Can you work these out from the drawing? Everything is in mm from the part's minimum corner. A direction names the side the tool comes from. Coordinates: 2 decimals unless noted, no trailing zeros. Loops run counter-clockwise (first coordinate to the right, second up) from the corner with the lowest first, then second, coordinate; pieces in that order, holes last.
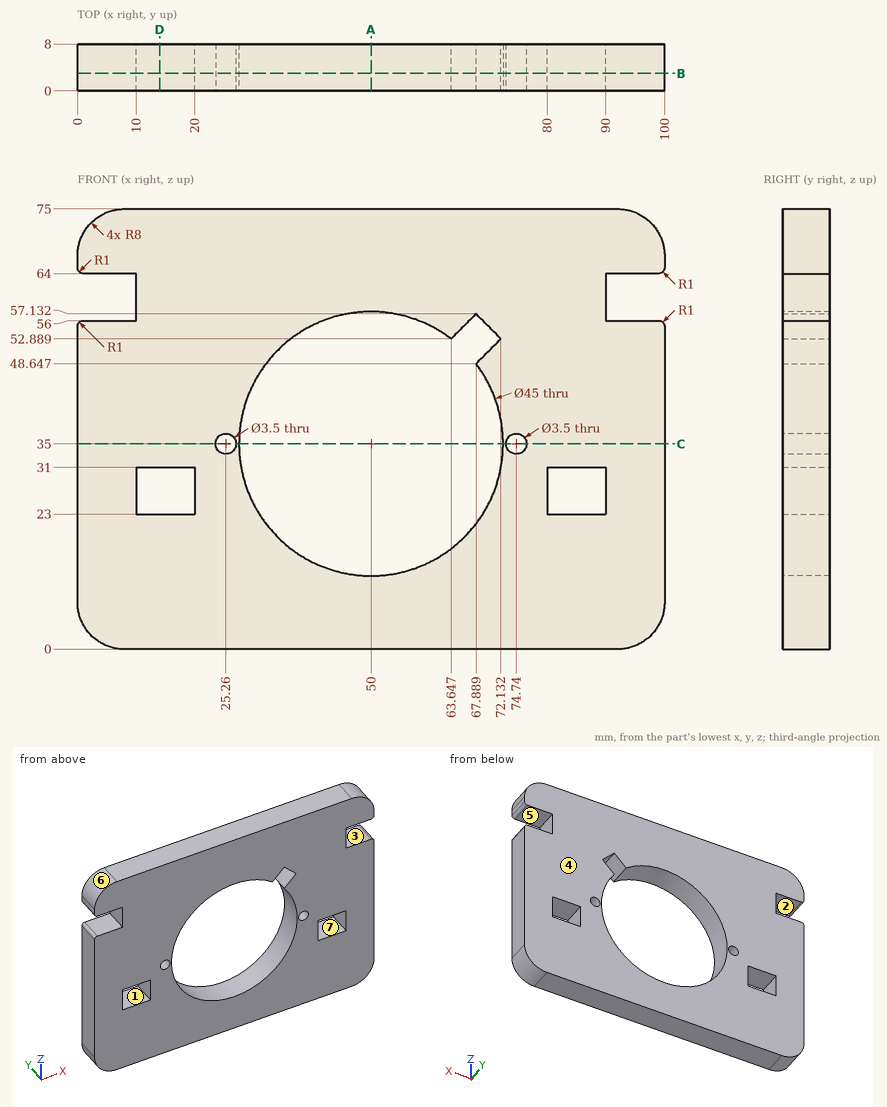
Item 1: On a 3-axis mill with a long thin cutter (end or side, diameter ignored), from which of +Z, -Z, +X, -X, +Y, -Y can I reach the whole of each face in a straight line? I mean the marked faces 1, 2 and 3. Say none if no direction works.
Results are:
face 1: +Y, -Y
face 2: -X, +Y, -Y
face 3: +X, +Y, -Y
Item 2: I need wall thicknesses on line 1 along X through (y, z) = (4.5, 35); line 2 along Z through (x, y) = (13.5, 7); line 3 along Z through (x, y) = (25.26, 4). Which ranges of each line are inside material? Lowest first, please.
Results are:
line 1: x = 0 to 23.51, 27.01 to 27.5, 72.5 to 72.99, 76.49 to 100
line 2: z = 0 to 23, 31 to 75
line 3: z = 0 to 33.25, 36.75 to 75
Item 3: Suppose I cut it at B-B, the plane y = 3. Count the separate pieces of the cut face and the enclosed holes in it, plus the area to 3 significant figures.
Results are:
separate pieces: 1
enclosed holes: 5
area: 5,480 mm2
Item 4: Suppose I cut it at D-D, the plane x = 14. Please give me the cut outline in (y, z), plus the area to 3 significant figures.
Results are:
outline: (0, 0) - (8, 0) - (8, 23) - (0, 23) - close; (0, 31) - (8, 31) - (8, 75) - (0, 75) - close
area: 536 mm2
Item 5: Suppose I cut it at A-A, the plane x = 50. Please give me the cut outline in (y, z), plus the area to 3 significant figures.
Results are:
outline: (0, 0) - (8, 0) - (8, 12.5) - (0, 12.5) - close; (0, 57.5) - (8, 57.5) - (8, 75) - (0, 75) - close
area: 240 mm2
Item 6: I'm going to push flat-ended pins straight in: P1, Ø2.5, axis at x = 7, y = 4.5, coming from the +Z side; P2, Ø2.5, axis at y = 2, z = 60, coming from the +X side; P3, Ø2.5, axis at y = 2.5, z = 62, coming from the -X side. Where does each tip first touch, or does it pass through?
Results are:
P1: stops at z = 75
P2: stops at x = 90
P3: stops at x = 10
Item 7: We'd pull the mould along Z, two halves only. Please class the marked faces 4, 5, 6 and 7: +Z half, -Z half, draft (parallel to the pull), parting line (faces both ways), or undercut.
Results are:
face 4: draft
face 5: undercut
face 6: +Z half
face 7: undercut
Item 8: Suppose I cut it at C-C, the plane z = 35. Please give me the cut outline in (x, y), plus the area to 3 significant figures.
Results are:
outline: (0, 0) - (23.51, 0) - (23.51, 8) - (0, 8) - close; (27.01, 0) - (27.5, 0) - (27.5, 8) - (27.01, 8) - close; (72.5, 0) - (72.99, 0) - (72.99, 8) - (72.5, 8) - close; (76.49, 0) - (100, 0) - (100, 8) - (76.49, 8) - close
area: 384 mm2
